from build123d import *

# Parameters (mm, degrees)
BOSS_EXTRUDE1_DEPTH             = 10
SKETCH2_R                       = 45
BOSS_EXTRUDE2_DEPTH             = 14
SKETCH3_R                       = 31.1
CUT_EXTRUDE1_DEPTH              = 21
F_4_0MM_DOWEL_HOLE1_D           = 4
F_4_0MM_DOWEL_HOLE1_CSINK_D     = 4.05
F_4_0MM_DOWEL_HOLE1_CSINK_ANGLE = 90
SKETCH11_R                      = 40
CUT_EXTRUDE2_DEPTH              = 5
SKETCH4_R                       = 24
CUT_EXTRUDE3_DEPTH              = 4
SKETCH12_R                      = 2
CUT_EXTRUDE5_DEPTH              = 4


with BuildPart() as part:
    # Sketch1 → Boss-Extrude1 (new body)
    with BuildSketch(Plane.XY):
        with BuildLine():
            Line((-42.5, 7.5), (-59.529404499, 7.5))
            ThreePointArc((-59.529404499, 7.5), (-60, 0), (-59.529404499, -7.5))
            Line((-59.529404499, -7.5), (-42.5, -7.5))
            Line((-42.5, -7.5), (-42.5, 7.5))
        make_face()
        with BuildLine():
            ThreePointArc((-7.5, 59.529404499), (-42.426406871, 42.426406871), (-59.529404499, 7.5))
            Line((-59.529404499, 7.5), (-42.5, 7.5))
            Line((-42.5, 7.5), (-42.5, -7.5))
            Line((-42.5, -7.5), (-59.529404499, -7.5))
            ThreePointArc((-59.529404499, -7.5), (-42.426406871, -42.426406871), (-7.5, -59.529404499))
            Line((-7.5, -59.529404499), (-7.5, -42.5))
            Line((-7.5, -42.5), (7.5, -42.5))
            Line((7.5, -42.5), (7.5, -59.529404499))
            ThreePointArc((7.5, -59.529404499), (42.426406871, -42.426406871), (59.529404499, -7.5))
            Line((59.529404499, -7.5), (42.5, -7.5))
            Line((42.5, -7.5), (42.5, 7.5))
            Line((42.5, 7.5), (59.529404499, 7.5))
            ThreePointArc((59.529404499, 7.5), (42.426406871, 42.426406871), (7.5, 59.529404499))
            Line((7.5, 59.529404499), (7.5, 42.5))
            Line((7.5, 42.5), (-7.5, 42.5))
            Line((-7.5, 42.5), (-7.5, 59.529404499))
        make_face()
        with BuildLine():
            ThreePointArc((7.5, 59.529404499), (0, 60), (-7.5, 59.529404499))
            Line((-7.5, 59.529404499), (-7.5, 42.5))
            Line((-7.5, 42.5), (7.5, 42.5))
            Line((7.5, 42.5), (7.5, 59.529404499))
        make_face()
        with BuildLine():
            Line((-7.5, 72.5), (-7.5, 59.529404499))
            ThreePointArc((-7.5, 59.529404499), (0, 60), (7.5, 59.529404499))
            Line((7.5, 59.529404499), (7.5, 72.5))
            Line((7.5, 72.5), (2.5, 77.5))
            Line((2.5, 77.5), (-2.5, 77.5))
            Line((-2.5, 77.5), (-7.5, 72.5))
        make_face()
        with BuildLine():
            Line((-59.529404499, 7.5), (-72.5, 7.5))
            Line((-72.5, 7.5), (-77.5, 2.5))
            Line((-77.5, 2.5), (-77.5, -2.5))
            Line((-77.5, -2.5), (-72.5, -7.5))
            Line((-72.5, -7.5), (-59.529404499, -7.5))
            ThreePointArc((-59.529404499, -7.5), (-60, 0), (-59.529404499, 7.5))
        make_face()
        with BuildLine():
            ThreePointArc((60, 0), (59.882235554, 3.757374753), (59.529404499, 7.5))
            Line((59.529404499, 7.5), (42.5, 7.5))
            Line((42.5, 7.5), (42.5, -7.5))
            Line((42.5, -7.5), (59.529404499, -7.5))
            ThreePointArc((59.529404499, -7.5), (59.882235554, -3.757374753), (60, 0))
        make_face()
        with BuildLine():
            Line((72.5, 7.5), (59.529404499, 7.5))
            ThreePointArc((59.529404499, 7.5), (59.882235554, 3.757374753), (60, 0))
            ThreePointArc((60, 0), (59.882235554, -3.757374753), (59.529404499, -7.5))
            Line((59.529404499, -7.5), (72.5, -7.5))
            Line((72.5, -7.5), (77.5, -2.5))
            Line((77.5, -2.5), (77.5, 2.5))
            Line((77.5, 2.5), (72.5, 7.5))
        make_face()
        with BuildLine():
            ThreePointArc((7.5, -59.529404499), (0, -60), (-7.5, -59.529404499))
            Line((-7.5, -59.529404499), (-7.5, -72.5))
            Line((-7.5, -72.5), (-2.5, -77.5))
            Line((-2.5, -77.5), (2.5, -77.5))
            Line((2.5, -77.5), (7.5, -72.5))
            Line((7.5, -72.5), (7.5, -59.529404499))
        make_face()
        with BuildLine():
            Line((-7.5, -42.5), (-7.5, -59.529404499))
            ThreePointArc((-7.5, -59.529404499), (0, -60), (7.5, -59.529404499))
            Line((7.5, -59.529404499), (7.5, -42.5))
            Line((7.5, -42.5), (-7.5, -42.5))
        make_face()
    extrude(amount=BOSS_EXTRUDE1_DEPTH)

    # Sketch2 → Boss-Extrude2 (add)
    with BuildSketch(Plane.XY.offset(10)):
        Circle(SKETCH2_R)
    extrude(amount=BOSS_EXTRUDE2_DEPTH)

    # Sketch3 → Cut-Extrude1 (cut)
    with BuildSketch(Plane.XY.offset(24)):
        Circle(SKETCH3_R)
    extrude(amount=-CUT_EXTRUDE1_DEPTH, mode=Mode.SUBTRACT)

    # Ø4.0mm Dowel Hole1 (through all)
    with Locations(Plane(origin=(0, 0, 0), x_dir=(-1, 0, 0), z_dir=(0, 0, -1))):
        with Locations((-70, 0), (0, 70), (70, 0), (0, -70)):
            CounterSinkHole(F_4_0MM_DOWEL_HOLE1_D / 2, F_4_0MM_DOWEL_HOLE1_CSINK_D / 2, counter_sink_angle=F_4_0MM_DOWEL_HOLE1_CSINK_ANGLE)

    # Sketch11 → Cut-Extrude2 (cut)
    with BuildSketch(Plane.XY.offset(24)):
        Circle(SKETCH11_R)
    extrude(amount=-CUT_EXTRUDE2_DEPTH, mode=Mode.SUBTRACT)

    # Sketch4 → Cut-Extrude3 (cut)
    with BuildSketch(Plane(origin=(0, 0, 0), x_dir=(-1, 0, 0), z_dir=(0, 0, -1))):
        Circle(SKETCH4_R)
    extrude(amount=-CUT_EXTRUDE3_DEPTH, mode=Mode.SUBTRACT)

    # Sketch12 → Cut-Extrude5 (cut)
    with BuildSketch(Plane(origin=(0, 0, 0), x_dir=(-1, 0, 0), z_dir=(0, 0, -1))):
        with Locations((27.5, 0)):
            Circle(SKETCH12_R)
        with Locations((0, -27.5)):
            Circle(SKETCH12_R)
        with Locations((-27.5, 0)):
            Circle(SKETCH12_R)
        with Locations((0, 27.5)):
            Circle(SKETCH12_R)
    extrude(amount=-CUT_EXTRUDE5_DEPTH, mode=Mode.SUBTRACT)


solid = part.part
CAD build for the part. Positions are in the model's coordinates, mm. A direction names the side the tool comes from. Round coordinates to 2 decimals unless told otherwise and drop trailing zeros. Loops run counter-clockwise (first coordinate to the right, second up) from the corner with the lowest first, then second, coordinate; pieces in that order, holes last.
(1) Drop flat-ended pins along their axis: pin 1 (4 mm diameter, centred on x = 40.5, y = -26.5, fed in from +Z); pin 2 (3 mm diameter, centred on x = -70, y = 0, fed in from +Z) (1 decimal); pin 3 (5 mm diameter, centred on x = -38, y = 14.5, fed in from -Z); pin 4 (2 mm diameter, centred on y = 10, z = 7, fed in from -X). Give the stop position or say it passes through.
(2) Cut at C-C (x = 0). State how many separate pieces and enclosed holes the cut face has, plus the area to 3 significant figures.
(3) Which spindle directions (+Z, -Z, +X, -X, +Y, -Y) get a long thin tool onto all of the face, cutting with end or side? Do faces 4 (the cylindrical face through (0.434, -29.452, 1.479)), 5 (the flat face through (7.5, -66, 5)), 6 (the flat face through (0, -46, 10)), 7 (the flat face through (-66, 7.5, 5)), 8 (the flat face through (75, 5, 5)). Say none if no direction does.
(4) Cut at A-A (x = -70). Give the cut face in (y, z) (3 decimals), plus the area to 3 significant figures.
(5) Cut at D-D (z = 15.75). Give the cut face in (x, y), plus the area to 3 significant figures.
(6) Wall check: line 1 along Y through (x, z) = (0, 3.5); line 2 along Y through (x, z) = (0, 1.15); line 3 along X through (y, z) = (-70, 3.25). Give the ranges that are in metal, low to high.
(7) Two-plate mould, pull along X, no slides. Class faces 1 (the cylindrical face through (25.592, 0.601, 1.479)), 2 (the cylindrical face through (42.03, -42.82, 4.93)), 3 (the cylindrical face through (20.765, -39.923, 16.902)): +X half, -X half, draft (parallel to the pull), parting line (faces both ways), or undercut.
Findings below:
1. pin 1: stops at z = 10
1. pin 2: passes through
1. pin 3: stops at z = 0
1. pin 4: stops at x = -59.32
2. separate pieces: 6
2. enclosed holes: 0
2. area: 1,170 mm2
3. face 4: +Z, -Z
3. face 5: +Z, -Z, +X, -Y
3. face 6: +Z
3. face 7: +Z, -Z, -X, +Y
3. face 8: +Z, -Z, +X, +Y
4. outline: (-7.5, 0) - (-2.025, 0) - (-2, 0.025) - (-2, 10) - (-7.5, 10) - close; (2, 0.025) - (2.025, 0) - (7.5, 0) - (7.5, 10) - (2, 10) - close
4. area: 110 mm2
5. outline: circle Ø90 at (0, 0); hole circle Ø62.2 at (0, 0)
5. area: 3,320 mm2
6. line 1: y = -77.5 to -72, -68 to -31.1, 31.1 to 68, 72 to 77.5
6. line 2: y = -77.5 to -72, -68 to -29.5, -25.5 to -24, 24 to 25.5, 29.5 to 68, 72 to 77.5
6. line 3: x = -7.5 to -2, 2 to 7.5
7. face 1: undercut
7. face 2: +X half
7. face 3: parting line
